from build123d import *

# Parameters (mm, degrees)
F0_W     = 50
F0_H     = 50
F1_DEPTH = 25
F3_DEPTH = 25


with BuildPart() as f1:
    # F0 (on Right) → F1 (new body)
    with BuildSketch(Plane.YZ):
        Rectangle(F0_W, F0_H)
    extrude(amount=F1_DEPTH)

    # F2 (on face) → F3 (cut)
    with BuildSketch(Plane.YZ.offset(25)):
        with BuildLine():
            ThreePointArc((8.73245, -14.845164), (-12.178559, -12.178559), (-14.845164, 8.73245))
            ThreePointArc((-14.845164, 8.73245), (-15.73245, 12.154836), (-19.154836, 11.26755))
            ThreePointArc((-19.154836, 11.26755), (-15.714093, -15.714093), (11.26755, -19.154836))
            ThreePointArc((11.26755, -19.154836), (12.154836, -15.73245), (8.73245, -14.845164))
        make_face()
    extrude(amount=-F3_DEPTH, mode=Mode.SUBTRACT)


solid = f1.part
CAD build for the part. Positions are in the model's coordinates, mm. Coordinates: 2 decimals unless noted, no trailing zeros. Order: outer loops, then holes, each group sorted by start corner. A loop starts at its lowest first (then second) coordinate and runs counter-clockwise, first axis right, second up.
Item 1: Band-saw the part on C-C on z = 0.5. List the corners of the cut face in (x, y).
Check sheet entries:
outline: (0, -25) - (25, -25) - (25, -22.22) - (0, -22.22) - close; (0, -17.22) - (25, -17.22) - (25, 25) - (0, 25) - close
Item 2: Two-plate mould, pull along Y, no slides. Class faces 1 (the face through (12, 0, -25)), 2 (the face through (12.68, -15.69, 12.13)), 3 (the face through (12, 25, 0)): +Y half, -Y half, draft (parallel to the pull), parting line (faces both ways), or undercut.
Check sheet entries:
face 1: draft
face 2: undercut
face 3: +Y half
Item 3: Band-saw the part on B-B on x = 4.5. List the corners of the cut face in (y, z), plus the area to 3 significant figures.
Check sheet entries:
outline: (-25, -25) - (25, -25) - (25, 25) - (-25, 25) - close; hole (-19.15, 11.27) arc R22.22 ccw to (11.27, -19.15) arc R2.5 ccw to (8.73, -14.85) arc R17.22 cw to (-14.85, 8.73) arc R2.5 ccw to start
area: 2,220 mm2
Item 4: Drill centre lines: L1, parallel to Y at x = 15, z = 0.5; L2, parallel to Z at x = 6, y = 8; L3, parallel to Y at x = 21.5, z = 6. Where is each one in solid material? Low to high.
Check sheet entries:
L1: y = -25 to -22.22, -17.22 to 25
L2: z = -25 to -20.73, -15.25 to 25
L3: y = -25 to -21.4, -16.14 to 25
Item 5: Band-saw the part on A-A on y = -11. List the corners of the cut face in (x, z), plus the area to 3 significant figures.
Check sheet entries:
outline: (0, -25) - (25, -25) - (25, -19.31) - (0, -19.31) - close; (0, -13.25) - (25, -13.25) - (25, 25) - (0, 25) - close
area: 1,100 mm2
